```python
from build123d import *

# Parameters (mm, degrees)
SKETCH1_R           = 6
SKETCH1_R_2         = 1.6
BOSS_EXTRUDE1_DEPTH = 10
SKETCH2_W           = 1.332407761
SKETCH2_H           = 7
SKETCH4_R           = 3.25
CUT_EXTRUDE1_DEPTH  = 3


with BuildPart() as part:
    # Sketch1 → Boss-Extrude1 (new body)
    with BuildSketch(Plane.XY):
        Circle(SKETCH1_R)
        Circle(SKETCH1_R_2, mode=Mode.SUBTRACT)
    extrude(amount=BOSS_EXTRUDE1_DEPTH)

    # Sketch2 → Cut-Revolve1 (revolve, cut)
    with BuildSketch(Plane(origin=(0, 0, 0), x_dir=(1, 0, 0), z_dir=(0, 1, 0))):
        with Locations((-5.666203881, -5)):
            Rectangle(SKETCH2_W, SKETCH2_H)
    revolve(axis=Axis((0, 0, 0), (0, 0, 1)), mode=Mode.SUBTRACT)

    # Sketch4 → Cut-Extrude1 (cut)
    with BuildSketch(Plane.XY.offset(10)):
        Circle(SKETCH4_R)
    extrude(amount=-CUT_EXTRUDE1_DEPTH, mode=Mode.SUBTRACT)


solid = part.part
```
Geometry check sheet. Reference: the model listing, model coordinates, mm. A direction names the side the tool comes from. Give positions to 0.01 mm unless a question says otherwise; leave off trailing zeros. Order: outer loops, then holes, each group sorted by start corner. A loop starts at its lowest first (then second) coordinate and runs counter-clockwise, first axis right, second up. Notation, with made-up numbers: (64.5, -21) - (78.5, -21) arc R13 ccw to (78.5, -7) - close; hole circle Ø1 at (-33, 40.25). An arc over 180 degrees is marked (long way). Answer in a Markdown table with one row per item. Add a question column.
Q1. Gauge pin test, flat ends, axial feed: pin 1 (3 mm diameter, centred on y = -2, z = 2.5, fed in from -X); pin 2 (5 mm diameter, centred on y = -4, z = 3, fed in from -X); pin 3 (1.5 mm diameter, centred on y = 0.5, z = 5.5, fed in from -X). Record the tip position at first contact, or that the pin passes through.
Q2. Tool access check on faces 5 (the flat face through (4, -4, 1.5)), 6 (the cylindrical face through (-2.579, -1.978, 8.521)), 7 (the cylindrical face through (-6, 0, 1)). Record the directions out of +Z, -Z, +X, -X, +Y, -Y that give a thin tool (end or side, any length) a straight path to the whole face; none if there is none.
Q3. Cross-section at A-A, the plane y = 0. Enter the section's corners in (x, z).
Q4. Material ranges on probe 1 along Z at (x, y) = (4, 4); probe 2 along Y at (x, z) = (0, 8.3); probe 3 along X at (y, z) = (0, 4.5), recorded low to high. Write a range as from..to.
Q5. Cross-section at D-D, the plane y = -3.5. Enter the section's corners in (x, z).
Q6. Mould release check, pull along Y, two halves, no side actions. Record for faces 1 (the flat face through (1.4, -1.4, 7)), 2 (the cylindrical face through (0.651, -4.957, 4.951)), 3 (the cylindrical face through (-1.27, -0.97, 3.45)), 4 (the flat face through (3, -3, 10)): pulls with the +Y half, pulls with the -Y half, needs draft (parallel to the pull), parting line crosses it, or undercut.
Q7. Cross-section at C-C, the plane z = 3.5. Enter the section's corners in (x, y).
Check values:
| question | item | result |
|---|---|---|
| 1 | pin 1 | stops at x = -5.93 |
| 1 | pin 2 | stops at x = -5.66 |
| 1 | pin 3 | stops at x = -5 |
| 2 | face 5 | none |
| 2 | face 6 | +Z |
| 2 | face 7 | +Z, -Z |
| 3 | outline | (-6, 0) - (-1.6, 0) - (-1.6, 7) - (-3.25, 7) - (-3.25, 10) - (-6, 10) - (-6, 8.5) - (-5, 8.5) - (-5, 1.5) - (-6, 1.5) - close; (1.6, 0) - (6, 0) - (6, 1.5) - (5, 1.5) - (5, 8.5) - (6, 8.5) - (6, 10) - (3.25, 10) - (3.25, 7) - (1.6, 7) - close |
| 4 | probe 1 | z = 0..1.5, 8.5..10 |
| 4 | probe 2 | y = -5..-3.25, 3.25..5 |
| 4 | probe 3 | x = -5..-1.6, 1.6..5 |
| 5 | outline | (-4.87, 0) - (4.87, 0) - (4.87, 1.5) - (3.57, 1.5) - (3.57, 8.5) - (4.87, 8.5) - (4.87, 10) - (-4.87, 10) - (-4.87, 8.5) - (-3.57, 8.5) - (-3.57, 1.5) - (-4.87, 1.5) - close |
| 6 | face 1 | undercut |
| 6 | face 2 | parting line crosses it |
| 6 | face 3 | undercut |
| 6 | face 4 | needs draft |
| 7 | outline | circle Ø10 at (0, 0); hole circle Ø3.2 at (0, 0) |
